Source: CAD feature listing. Evaluate the final solid. Frame: model axes, mm. Coordinates: 2 decimals unless noted, no trailing zeros. Write each loop counter-clockwise with the first axis right and the second up, starting at its lowest first coordinate (ties: lowest second). Pieces come first, ordered by that corner, then holes. Notation, with made-up numbers: (-19, 35.5) - (-6, 35.5) arc R29 ccw to (-6, 65.5) - close; hole circle Ø8 at (-22.5, 41). An arc over 180 degrees is marked (long way). One line per item, written item: value.
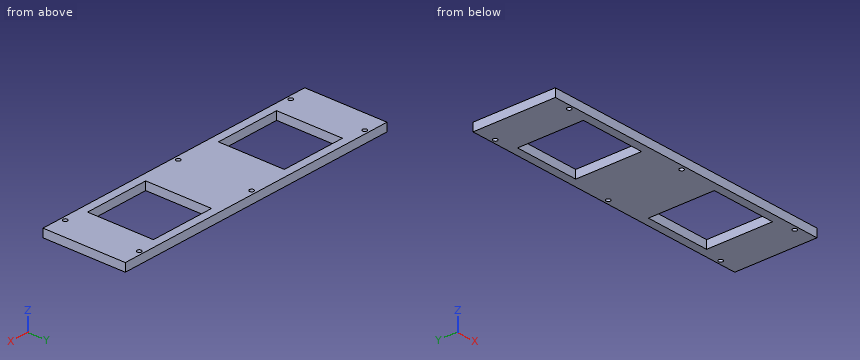
from build123d import *

# Parameters (mm, degrees)
F0_W     = 540
F0_H     = 150
F0_R     = 4
F0_W_2   = 120
F0_H_2   = 120
F1_DEPTH = 15


with BuildPart() as f1:
    # F0 (on Top) → F1 (new body)
    with BuildSketch(Plane.XY):
        with Locations((270, -75)):
            Rectangle(F0_W, F0_H)
        with Locations((37.449412, -142.458765)):
            Circle(F0_R, mode=Mode.SUBTRACT)
        with Locations((270, -141.832436)):
            Circle(F0_R, mode=Mode.SUBTRACT)
        with Locations((502.550588, -142.458765)):
            Circle(F0_R, mode=Mode.SUBTRACT)
        with Locations((134.932024, -75)):
            Rectangle(F0_W_2, F0_H_2, mode=Mode.SUBTRACT)
        with Locations((37.449412, -7.541235)):
            Circle(F0_R, mode=Mode.SUBTRACT)
        with Locations((405.067976, -75)):
            Rectangle(F0_W_2, F0_H_2, mode=Mode.SUBTRACT)
        with Locations((270, -8.167564)):
            Circle(F0_R, mode=Mode.SUBTRACT)
        with Locations((502.550588, -7.541235)):
            Circle(F0_R, mode=Mode.SUBTRACT)
    extrude(amount=F1_DEPTH)


solid = f1.part
1) Section query C-C on z = 2.75. State how many separate pieces and enclosed holes the cut face has, then the cut area to 3 significant figures.
Values found:
separate pieces: 1
enclosed holes: 8
area: 51,900 mm2
2) Section query B-B on y = -42. Output: boundary loops of the cut face in (x, z), then the cut area to 3 significant figures.
Values found:
outline: (0, 0) - (74.93, 0) - (74.93, 15) - (0, 15) - close; (194.93, 0) - (345.07, 0) - (345.07, 15) - (194.93, 15) - close; (465.07, 0) - (540, 0) - (540, 15) - (465.07, 15) - close
area: 4,500 mm2
3) Section query A-A on x = 89. Output: boundary loops of the cut face in (y, z).
Values found:
outline: (-150, 0) - (-135, 0) - (-135, 15) - (-150, 15) - close; (-15, 0) - (0, 0) - (0, 15) - (-15, 15) - close
4) Material intervals for line 1 (X direction, y = -58.5, z = 12.25); line 2 (Y direction, x = 270, z = 6.25); line 3 (Y direction, x = 424, z = 9.75), sorted ascending.
Values found:
line 1: 0 to 74.93, 194.93 to 345.07, 465.07 to 540
line 2: -150 to -145.83, -137.83 to -12.17, -4.17 to 0
line 3: -150 to -135, -15 to 0
